Can you work these out from the model? Positions are in its coordinate system, mm. A direction names the side the tool comes from. Round coordinates to 2 decimals unless told otherwise and drop trailing zeros. Order: outer loops, then holes, each group sorted by start corner. A loop starts at its lowest first (then second) coordinate and runs counter-clockwise, first axis right, second up. Notation, with made-up numbers: (-33, -7.5) - (-14, -7.5) arc R9 ccw to (-14, 2.5) - close; hole circle Ø9 at (-33, 20.25). An arc over 180 degrees is marked (long way). Write item = value, one per line.
from build123d import *

# Parameters (mm, degrees)
BOSS_EXTRUDE1_DEPTH = 1.65
FILLET1_R           = 2
FILLET2_R           = 2
FILLET3_R           = 1.5


with BuildPart() as part:
    # Sketch1 → Boss-Extrude1 (new body)
    with BuildSketch(Plane(origin=(0, 0, 0), x_dir=(1, 0, 0), z_dir=(0, 1, 0))):
        Polygon((-41.448800006, 34.091704203), (-34.091704203, 41.448800006), (34.091704203, 41.448800006), (41.448800006, 34.091704203), (41.448800006, -34.091704203), (34.091704203, -41.448800006), (-34.091704203, -41.448800006), (-41.448800006, -34.091704203), align=None)
        Polygon((-39.798800006, 33.408251825), (-33.408251825, 39.798800006), (-29.292890359, 39.798800006), (-39.798800006, 29.292890359), align=None, mode=Mode.SUBTRACT)
        Polygon((-33.408251825, -39.798800006), (-29.292890359, -39.798800006), (-39.798800006, -29.292890359), (-39.798800006, -33.408251825), align=None, mode=Mode.SUBTRACT)
        Polygon((39.798800006, -33.408251825), (39.798800006, -29.292890359), (29.292890359, -39.798800006), (33.408251825, -39.798800006), align=None, mode=Mode.SUBTRACT)
        Polygon((33.408251825, 39.798800006), (39.798800006, 33.408251825), (39.798800006, 29.292890359), (29.292890359, 39.798800006), align=None, mode=Mode.SUBTRACT)
        Polygon((-39.798800006, 26.959437981), (-26.959437981, 39.798800006), (26.959437981, 39.798800006), (39.798800006, 26.959437981), (39.798800006, -26.959437981), (26.959437981, -39.798800006), (-26.959437981, -39.798800006), (-39.798800006, -26.959437981), align=None, mode=Mode.SUBTRACT)
    extrude(amount=BOSS_EXTRUDE1_DEPTH)

    # Fillet1
    fillet1_edges = [part.edges().sort_by_distance(p)[0] for p in [
        (-41.448800006, 0.825, -34.091704203),
        (-34.091704203, 0.825, -41.448800006),
        (-39.798800006, 0.825, -26.959437981),
        (-26.959437981, 0.825, -39.798800006),
    ]]
    fillet(fillet1_edges, radius=FILLET1_R)

    # Fillet2
    fillet2_edges = [part.edges().sort_by_distance(p)[0] for p in [
        (34.091704203, 0.825, -41.448800006),
        (41.448800006, 0.825, -34.091704203),
        (41.448800006, 0.825, 34.091704203),
        (34.091704203, 0.825, 41.448800006),
        (-34.091704203, 0.825, 41.448800006),
        (-41.448800006, 0.825, 34.091704203),
        (-39.798800006, 0.825, 26.959437981),
        (-26.959437981, 0.825, 39.798800006),
        (26.959437981, 0.825, 39.798800006),
        (39.798800006, 0.825, 26.959437981),
        (39.798800006, 0.825, -26.959437981),
        (26.959437981, 0.825, -39.798800006),
    ]]
    fillet(fillet2_edges, radius=FILLET2_R)

    # Fillet3
    fillet3_edges = [part.edges().sort_by_distance(p)[0] for p in [
        (-39.798800006, 0.825, -29.292890359),
        (-29.292890359, 0.825, -39.798800006),
        (29.292890359, 0.825, -39.798800006),
        (39.798800006, 0.825, -29.292890359),
        (39.798800006, 0.825, 29.292890359),
        (29.292890359, 0.825, 39.798800006),
        (-29.292890359, 0.825, 39.798800006),
        (-39.798800006, 0.825, 29.292890359),
    ]]
    fillet(fillet3_edges, radius=FILLET3_R)


solid = part.part
(1) If we section it at B-B (z = 19): Write out the boundary of the cut face in (x, y), plus the area to 4 significant figures.
Computed:
outline = (-41.45, 0) - (-39.8, 0) - (-39.8, 1.65) - (-41.45, 1.65) - close; (39.8, 0) - (41.45, 0) - (41.45, 1.65) - (39.8, 1.65) - close
area = 5.445 mm^2
(2) On a 3-axis mill with a long thin cutter (end or side, diameter ignored), from which of +Z, -Z, +X, -X, +Y, -Y can I reach the whole of each face in a straight line? I mean faces 1 (the face through (-37.81, 0.81, -37.73)), 2 (the face through (-36.648, 0.813, -36.559)). Say none if no direction works.
Computed:
face_1 = -Z, -X, +Y, -Y
face_2 = +Y, -Y
(3) If I drill on line 1 (X direction, y = 1.45, z = -25); line 2 (X direction, y = 0.5, z = 37), over which ranges is the centre line in solid material (lowest first)? Write a range as from..to.
Computed:
line_1 = -41.45..-39.8, 39.8..41.45
line_2 = -38.54..-36.21, -32.09..-29.76, 29.76..32.09, 36.21..38.54
(4) If we section it at C-C (y = 1): State how many separate pieces and enclosed holes the cut face has, plus the area to 3 significant figures.
Computed:
separate_pieces = 1
enclosed_holes = 5
area = 641 mm^2
(5) Thinking about a two-plate mould opening in Z: for faces 3 (the face through (-34.51, 0.81, 34.58)), 4 (the face through (-37.73, 0.81, 37.81)), 5 (the face through (9, 1.65, -40)), which applies, +Z half, -Z half, draft (parallel to the pull), parting line (faces both ways), or undercut?
Computed:
face_3 = undercut
face_4 = +Z half
face_5 = draft
(6) If we section it at A-A (x = 13.5): Write out the boundary of the cut face in (y, z).
Computed:
outline = (0, -41.45) - (1.65, -41.45) - (1.65, -39.8) - (0, -39.8) - close; (0, 39.8) - (1.65, 39.8) - (1.65, 41.45) - (0, 41.45) - close
